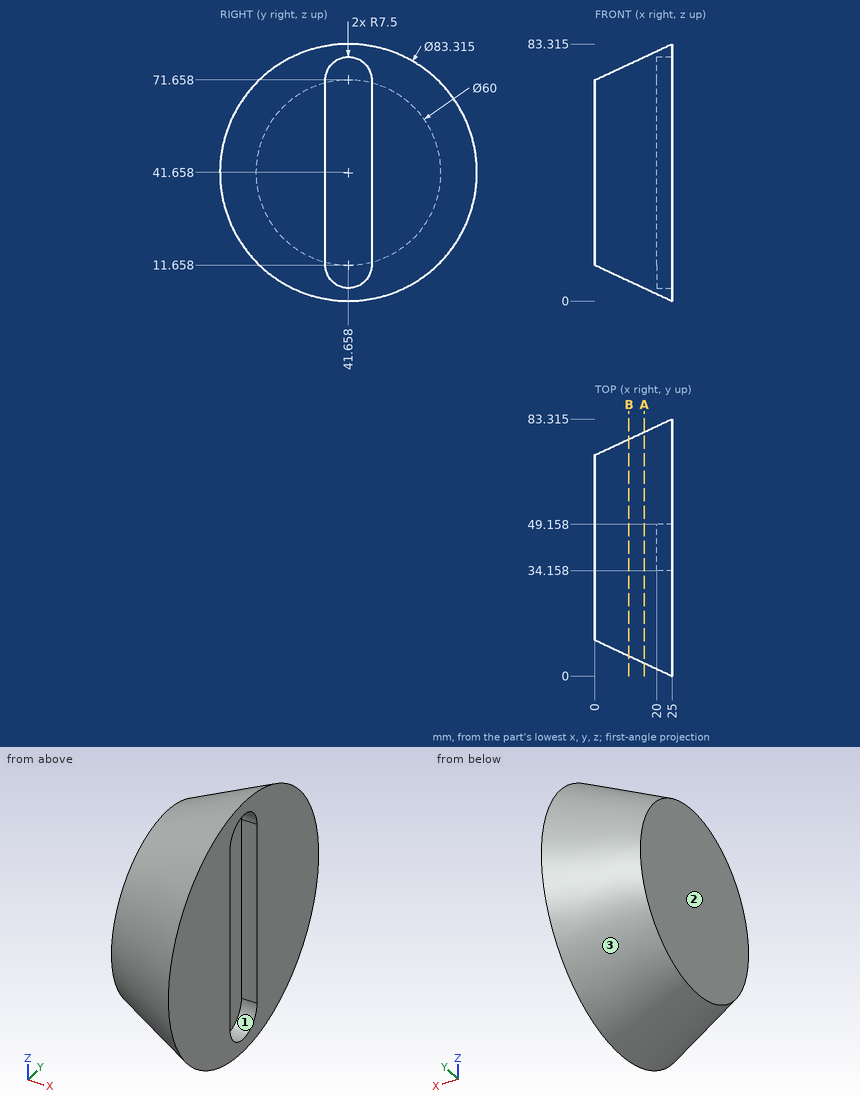
Part print with two shaded views. Sizes in mm from the minimum x, y, z corner. Give positions to 0.01 mm unless a question says otherwise; leave off trailing zeros. Order: outer loops, then holes, each group sorted by start corner. A loop starts at its lowest first (then second) coordinate and runs counter-clockwise, first axis right, second up.
1) Pin check, flat tips, straight feed: pin 1 (3 mm diameter, centred on y = 11, z = 36.5, fed in from -X); pin 2 (4 mm diameter, centred on x = 11.5, y = 21, fed in from +Z); pin 3 (5 mm diameter, centred on x = 4.5, z = 62, fed in from +Y); pin 4 (2 mm diameter, centred on x = 14, z = 30.5, fed in from +Y). Stop position of each tip, or through.
2) Mould opens along Z. For the marked faces 1, 2 and 3 say: +Z half, -Z half, draft (parallel to the pull), parting line (faces both ways), or undercut.
3) Saw through at B-B, the plane x = 11. Write the cut outline in (y, z), then the cut area to 3 significant figures.
4) Saw through at A-A, the plane x = 16. Write the cut outline in (y, z), then the cut area to 3 significant figures.
5) Wall check: probe 1 along X at (y, z) = (43, 70); probe 2 along Y at (x, z) = (21.25, 5) (1 decimal); probe 3 along Z at (x, y) = (14, 37.5). Give the ranges that are in metal, low to high.
Computed:
1. pin 1: stops at x = 0
1. pin 2: stops at z = 72.11
1. pin 3: stops at y = 68.85
1. pin 4: stops at y = 77.02
2. face 1: undercut
2. face 2: draft
2. face 3: parting line
3. outline: circle Ø70.26 at (41.66, 41.66)
3. area: 3,880 mm2
4. outline: circle Ø74.92 at (41.66, 41.66)
4. area: 4,410 mm2
5. probe 1: x = 0 to 20
5. probe 2: y = 25.9 to 38.2, 45.1 to 57.4
5. probe 3: z = 5.37 to 77.95
